Autodesk Inventor part; units mm, degrees
ref_plane "YZ Plane" through (0, 0, 0) normal (1, 0, 0) x (0, 1, 0)
ref_plane "XZ Plane" through (0, 0, 0) normal (0, 1, 0) x (-1, 0, 0)
ref_plane "XY Plane" through (0, 0, 0) normal (0, 0, 1) x (1, 0, 0)
sketch "Sketch1" plane through (0, 0, 0) normal (0, 1, 0) x (-1, 0, 0)
  line L0 (317.7202, 61.6798) -> (30.3202, 61.6798)
  line L1 (317.7202, 264.8798) -> (317.7202, 61.6798)
  line L2 (30.3202, 264.8798) -> (317.7202, 264.8798)
  line L3 (30.3202, 61.6798) -> (30.3202, 264.8798)
  arc A0 (0.0202, 15.9798) -> (16.0202, -0.0202) centre (16.0202, 15.9798) ccw
  line L4 (0.0202, 15.9798) -> (0.0202, 281.8798)
  arc A1 (16.0202, 297.8798) -> (0.0202, 281.8798) centre (16.0202, 281.8798) ccw
  line L5 (16.0202, 297.8798) -> (332.0202, 297.8798)
  arc A2 (348.0202, 281.8798) -> (332.0202, 297.8798) centre (332.0202, 281.8798) ccw
  line L6 (348.0202, 281.8798) -> (348.0202, 15.9798)
  arc A3 (332.0202, -0.0202) -> (348.0202, 15.9798) centre (332.0202, 15.9798) ccw
  line L7 (332.0202, -0.0202) -> (16.0202, -0.0202)
  arc A4 (21.2952, 6.4798) -> (25.0452, 6.4798) centre (23.1702, 6.4798) ccw
  line L8 (25.0452, 10.4798) -> (25.0452, 6.4798)
  arc A5 (25.0452, 10.4798) -> (21.2952, 10.4798) centre (23.1702, 10.4798) ccw
  line L9 (21.2952, 6.4798) -> (21.2952, 10.4798)
  arc A6 (52.2952, 6.4798) -> (56.0452, 6.4798) centre (54.1702, 6.4798) ccw
  line L10 (56.0452, 10.4798) -> (56.0452, 6.4798)
  arc A7 (56.0452, 10.4798) -> (52.2952, 10.4798) centre (54.1702, 10.4798) ccw
  line L11 (52.2952, 6.4798) -> (52.2952, 10.4798)
  arc A8 (21.2952, 37.4798) -> (25.0452, 37.4798) centre (23.1702, 37.4798) ccw
  line L12 (25.0452, 41.4798) -> (25.0452, 37.4798)
  arc A9 (25.0452, 41.4798) -> (21.2952, 41.4798) centre (23.1702, 41.4798) ccw
  line L13 (21.2952, 37.4798) -> (21.2952, 41.4798)
  arc A10 (52.2952, 37.4798) -> (56.0452, 37.4798) centre (54.1702, 37.4798) ccw
  line L14 (56.0452, 41.4798) -> (56.0452, 37.4798)
  arc A11 (56.0452, 41.4798) -> (52.2952, 41.4798) centre (54.1702, 41.4798) ccw
  line L15 (52.2952, 37.4798) -> (52.2952, 41.4798)
  arc A12 (26.6702, 21.9798) -> (50.6702, 21.9798) centre (38.6702, 21.9798) ccw
  line L16 (50.6702, 25.9798) -> (50.6702, 21.9798)
  arc A13 (50.6702, 25.9798) -> (26.6702, 25.9798) centre (38.6702, 25.9798) ccw
  line L17 (26.6702, 21.9798) -> (26.6702, 25.9798)
  arc A14 (291.9952, 6.4798) -> (295.7452, 6.4798) centre (293.8702, 6.4798) ccw
  line L18 (295.7452, 10.4798) -> (295.7452, 6.4798)
  arc A15 (295.7452, 10.4798) -> (291.9952, 10.4798) centre (293.8702, 10.4798) ccw
  line L19 (291.9952, 6.4798) -> (291.9952, 10.4798)
  arc A16 (322.9952, 6.4798) -> (326.7452, 6.4798) centre (324.8702, 6.4798) ccw
  line L20 (326.7452, 10.4798) -> (326.7452, 6.4798)
  line L21 (322.9952, 6.4798) -> (322.9952, 10.4798)
  arc A17 (322.9952, 37.4798) -> (326.7452, 37.4798) centre (324.8702, 37.4798) ccw
  line L22 (326.7452, 41.4798) -> (326.7452, 37.4798)
  arc A18 (326.7452, 41.4798) -> (322.9952, 41.4798) centre (324.8702, 41.4798) ccw
  line L23 (322.9952, 37.4798) -> (322.9952, 41.4798)
  arc A19 (291.9952, 37.4798) -> (295.7452, 37.4798) centre (293.8702, 37.4798) ccw
  line L24 (295.7452, 41.4798) -> (295.7452, 37.4798)
  arc A20 (295.7452, 41.4798) -> (291.9952, 41.4798) centre (293.8702, 41.4798) ccw
  line L25 (291.9952, 37.4798) -> (291.9952, 41.4798)
  arc A21 (297.3702, 21.9798) -> (321.3702, 21.9798) centre (309.3702, 21.9798) ccw
  line L26 (321.3702, 25.9798) -> (321.3702, 21.9798)
  arc A22 (321.3702, 25.9798) -> (297.3702, 25.9798) centre (309.3702, 25.9798) ccw
  line L27 (297.3702, 21.9798) -> (297.3702, 25.9798)
  circle A23 centre (50.2702, 272.8798) radius 1
  circle A24 centre (38.6702, 287.8798) radius 1
  circle A25 centre (309.3702, 287.8798) radius 1
  circle A26 centre (297.7702, 272.8798) radius 1
  circle A27 centre (25.9077, 270.3798) radius 1
  circle A28 centre (66.9077, 270.3798) radius 1
  circle A29 centre (174.0202, 270.3798) radius 1
  circle A30 centre (281.1327, 270.3798) radius 1
  circle A31 centre (322.1327, 270.3798) radius 1
  circle A32 centre (322.1327, 56.1798) radius 1
  circle A33 centre (281.1327, 56.1798) radius 1
  circle A34 centre (174.0202, 56.1798) radius 1
  circle A35 centre (66.9077, 56.1798) radius 1
  circle A36 centre (25.9077, 56.1798) radius 1
  arc A37 (326.7452, 10.4798) -> (322.9952, 10.4798) centre (324.8702, 10.4798) ccw
  point P0 (0, 0)
extrude "Extrusion1" add sketch "Sketch1" along normal blind 4.7625
properties part number "core xy plate"
Work out the finished part from the listing and answer in its coordinate system (mm). A direction names the side the tool comes from. Give positions to 0.01 mm unless a question says otherwise; leave off trailing zeros. Loops run counter-clockwise (first coordinate to the right, second up) from the corner with the lowest first, then second, coordinate; pieces in that order, holes last. Notation, with made-up numbers: (2.5, -10) -> (30.5, -10) arc R26 ccw to (30.5, 28) -> close; hole circle Ø5 at (-30.5, 3). An arc over 180 degrees is marked (long way). Use a Markdown table: item, result. Add a question column.
1. Section B-B on z = 153.5 is taken. Determine the outline of the cut face in (x, y).
2. Flat-ended cylindrical pins translate along their axes: pin 1 Ø1.2 at (x, z) = (-281.13, 270.38) entering from -Y; pin 2 Ø1.2 at (y, z) = (1.5, 8) entering from -X; pin 3 Ø2 at (y, z) = (3.5, 8.5) entering from +X. Find the tip coordinate at first contact, or state that the pin passes through.
3. Section C-C on y = 1.4 is taken. State how many separate pieces and enclosed holes the cut face has, and give its area (3 significant figures).
4. Find the intervals of material crossed by probe 1 along X at (y, z) = (4.65, 22); probe 2 along X at (y, z) = (3.5, 40); probe 3 along X at (y, z) = (1.65, 128), in increasing order.
5. Section A-A on x = -183.5 is taken. Determine the outline of the cut face in (y, z).
6. For faces 4 (the flat face through (-172, 0, 52)), 5 (the cylindrical face through (-38.406, 2.348, 37.977)), determine the directions among +Z, -Z, +X, -X, +Y, -Y from which every point of the face is accessible in a straight line to the end or side of a thin tool.
7. Determine the mould class of faces 1 (the cylindrical face through (-4.583, 2.348, 293.068)), 2 (the cylindrical face through (-343.458, 2.348, 4.791)), 3 (the cylindrical face through (-309.106, 2.348, 37.977)) for opening direction X: released by +X, released by -X, zero draft, split by the parting line, or undercut.
Results below:
| question | item | result |
|---|---|---|
| 1 | outline | (-348.02, 0) -> (-317.72, 0) -> (-317.72, 4.76) -> (-348.02, 4.76) -> close; (-30.32, 0) -> (-0.02, 0) -> (-0.02, 4.76) -> (-30.32, 4.76) -> close |
| 2 | pin 1 | passes through |
| 2 | pin 2 | stops at x = -346.22 |
| 2 | pin 3 | stops at x = -1.39 |
| 3 | separate pieces | 1 |
| 3 | enclosed holes | 25 |
| 3 | area | 43,700 mm^2 |
| 4 | probe 1 | x = -348.02 to -321.37, -297.37 to -50.67, -26.67 to -0.02 |
| 4 | probe 2 | x = -348.02 to -326.75, -323 to -295.75, -292 to -56.05, -52.3 to -25.05, -21.3 to -0.02 |
| 4 | probe 3 | x = -348.02 to -317.72, -30.32 to -0.02 |
| 5 | outline | (0, -0.02) -> (4.76, -0.02) -> (4.76, 61.68) -> (0, 61.68) -> close; (0, 264.88) -> (4.76, 264.88) -> (4.76, 297.88) -> (0, 297.88) -> close |
| 6 | face 4 | +Z, -Z, +X, -X, -Y |
| 6 | face 5 | +Y, -Y |
| 7 | face 1 | released by +X |
| 7 | face 2 | released by -X |
| 7 | face 3 | undercut |
